Design review of the part shown in the three views and the two pictorial views. Dimensions are in mm from the part's minimum x, y and z. Round coordinates to 2 decimals unless told otherwise and drop trailing zeros. Order: outer loops, then holes, each group sorted by start corner. A loop starts at its lowest first (then second) coordinate and runs counter-clockwise, first axis right, second up. Notation, with made-up numbers: M 5.25,1.5 L 26.25,1.5 A9 cw 26.25,8.5 Z; hole C 70.5,0.5 d7. An arc over 180 degrees is marked long. Write item = value, one per line. Start each with the question number.
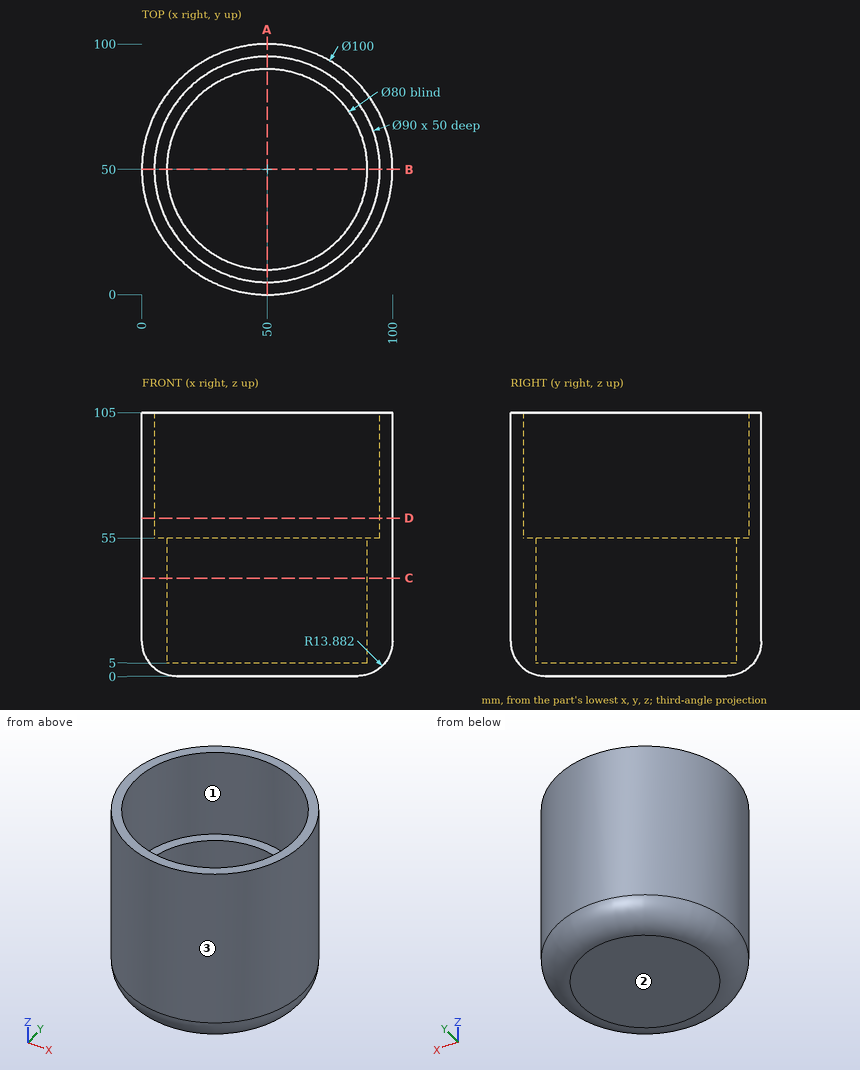
(1) We need section C-C, the plane z = 39. Write out the cut boundary in (x, y), then the cut area to 3 significant figures.
(2) We need section A-A, the plane x = 50. Write out the cut boundary in (y, z).
(3) Insertion check: pin 1 (1.5 mm diameter, centred on x = 78.5, z = 26.5, fed in from -Y); pin 2 (1.5 mm diameter, centred on x = 33.5, z = 24.5, fed in from -Y) (1 decimal); pin 3 (2 mm diameter, centred on y = 76, z = 56, fed in from -X). Each pin has a flat end and moves straight along its axis. Give the tip position at first contact, or say it passes through.
(4) For line 1 along Y through (x, z) = (50, 86.5); line 2 along X through (y, z) = (51.5, 26); line 3 along Z through (x, y) = (28, 21), list the stretches that pass through material, from the lowest coordinate up.
(5) Draft analysis for pull direction X (two halves, no side actions). For the marked faces 1, 2 and 3, state which applies: released by +X, released by -X, zero draft, split by the parting line, or undercut.
(6) We need section D-D, the plane z = 63. Write out the cut boundary in (x, y), then the cut area to 3 significant figures.
Values:
q1.outline = C 50,50 d100; hole C 50,50 d80
q1.area = 2,830 mm²
q2.outline = M 0,13.88 A13.88 ccw 13.88,0 L 86.12,0 A13.88 ccw 100,13.88 L 100,105 L 95,105 L 95,55 L 90,55 L 90,5 L 10,5 L 10,55 L 5,55 L 5,105 L 0,105 Z
q3.pin_1 = 8.41
q3.pin_2 = 2.5
q3.pin_3 = 6.7
q4.line_1 = 0 to 5, 95 to 100
q4.line_2 = 0.02 to 10.03, 89.97 to 99.98
q4.line_3 = 0 to 5
q5.face_1 = undercut
q5.face_2 = zero draft
q5.face_3 = split by the parting line
q6.outline = C 50,50 d100; hole C 50,50 d90
q6.area = 1,490 mm²
